```python
from build123d import *

# Parameters (mm, degrees)
SKETCH1_R               = 101.6
BOSS_EXTRUDE1_DEPTH     = 76.2
CUT_EXTRUDE7_DEPTH      = 163.639355631
CUT_EXTRUDE7_DEPTH_BACK = 163.639355631


with BuildPart() as part:
    # Sketch1 → Boss-Extrude1 (new body)
    with BuildSketch(Plane.XY):
        with Locations(Location((0, 0, 0), (0, 0, 180))):
            Circle(SKETCH1_R)
    extrude(amount=BOSS_EXTRUDE1_DEPTH)

    # Sketch2 → Cut-Extrude7 (cut, two sides: drawn at the far end of the back side and taken through both)
    with BuildSketch(Plane.XY.offset(76.2).offset(-CUT_EXTRUDE7_DEPTH_BACK)):
        with BuildLine():
            ThreePointArc((-55.703026842, -24.462175809), (-80.165202651, 0), (-55.703026842, 24.462175809))
            Line((-55.703026842, 24.462175809), (-55.703026842, -24.462175809))
        make_face()
        with BuildLine():
            Line((55.703026842, 24.462175809), (55.703026842, -24.462175809))
            ThreePointArc((55.703026842, -24.462175809), (80.165202651, 0), (55.703026842, 24.462175809))
        make_face()
    extrude(amount=CUT_EXTRUDE7_DEPTH + CUT_EXTRUDE7_DEPTH_BACK, mode=Mode.SUBTRACT)


solid = part.part
```
Work out the finished part from the listing and answer in its coordinate system (mm). A direction names the side the tool comes from. Round coordinates to 2 decimals unless told otherwise and drop trailing zeros. Order: outer loops, then holes, each group sorted by start corner. A loop starts at its lowest first (then second) coordinate and runs counter-clockwise, first axis right, second up.
Q1. Given pin 1 Ø1 at (x, y) = (-44, -34) entering from -Z; pin 2 Ø2 at (x, z) = (42.5, 56) entering from -Y; pin 3 Ø12 at (x, z) = (-69, 47) entering from +Y; pin 4 Ø2 at (x, z) = (-22.5, 25) entering from -Y, each flat-ended and moving along its own axis, determine where each tip first touches the part or whether it passes through.
Solution:
pin 1: stops at z = 0
pin 2: stops at y = -92.74
pin 3: stops at y = 79.71
pin 4: stops at y = -99.3
Q2. A cutting plane is placed at A-A, the plane y = 0. Determine the outline of the cut face in (x, z).
Solution:
outline: (-101.6, 0) - (-80.17, 0) - (-80.17, 76.2) - (-101.6, 76.2) - close; (-55.7, 0) - (55.7, 0) - (55.7, 76.2) - (-55.7, 76.2) - close; (80.17, 0) - (101.6, 0) - (101.6, 76.2) - (80.17, 76.2) - close
Q3. A tool of negligible diameter and unlimited length cuts with its end or side. For faces 1 (the flat face through (1, -1, 0)), 2 (the flat face through (-55.703, 0, 38)), from which of +Z, -Z, +X, -X, +Y, -Y can it reach the whole face along a straight path? Write none if from no direction.
Solution:
face 1: -Z, +X, -X, +Y, -Y
face 2: +Z, -Z
Q4. Find the intervals of material crossed by line 1 along X through (y, z) = (15, 42); line 2 along X through (y, z) = (2, 27.5); line 3 along Y through (x, z) = (-58, 8), in increasing order.
Solution:
line 1: x = -100.49 to -75.03, -55.7 to 55.7, 75.03 to 100.49
line 2: x = -101.58 to -80.08, -55.7 to 55.7, 80.08 to 101.58
line 3: y = -83.42 to -24.35, 24.35 to 83.42
Q5. A cutting plane is placed at D-D, the plane x = -61. Determine the outline of the cut face in (y, z), then the cut area to 3 significant figures.
Solution:
outline: (-81.25, 0) - (-23.88, 0) - (-23.88, 76.2) - (-81.25, 76.2) - close; (23.88, 0) - (81.25, 0) - (81.25, 76.2) - (23.88, 76.2) - close
area: 8,740 mm2
Q6. A cutting plane is placed at C-C, the plane z = 34. Determine the outline of the cut face in (x, y), then the cut area to 3 significant figures.
Solution:
outline: circle Ø203.2 at (0, 0); hole (-55.7, -24.46) - (-55.7, 24.46) arc R24.46 ccw to start; hole (55.7, -24.46) arc R24.46 ccw to (55.7, 24.46) - close
area: 30,500 mm2
Q7. The mould has two halves that part along Y. Classify faces 3 (the flat face through (55.703, 0, 38)), 4 (the cylindrical face through (-46.88, 90.14, 37.57)), 5 (the flat face through (1, -1, 76.2)), 6 (the cylindrical face through (-80.16, -0.54, 37.57)): pulls with the +Y half, pulls with the -Y half, needs draft (parallel to the pull), parting line crosses it, or undercut.
Solution:
face 3: undercut
face 4: parting line crosses it
face 5: needs draft
face 6: undercut
Q8. A cutting plane is placed at B-B, the plane x = 58.5. Determine the outline of the cut face in (y, z), then the cut area to 3 significant figures.
Solution:
outline: (-83.07, 0) - (-24.3, 0) - (-24.3, 76.2) - (-83.07, 76.2) - close; (24.3, 0) - (83.07, 0) - (83.07, 76.2) - (24.3, 76.2) - close
area: 8,960 mm2
